```python
from build123d import *

# Parameters (mm, degrees)
SKETCH1_R           = 2.5
BOSS_EXTRUDE1_DEPTH = 3
SKETCH2_R           = 1.5
BOSS_EXTRUDE2_DEPTH = 30
CHAMFER1_SIZE       = 0.3
FILLET1_R           = 0.4
CUT_EXTRUDE1_DEPTH  = 1.5


with BuildPart() as part:
    # Sketch1 → Boss-Extrude1 (new body)
    with BuildSketch(Plane(origin=(0, 0, 0), x_dir=(1, 0, 0), z_dir=(0, 1, 0))):
        with Locations(Location((0, 0, 0), (0, 0, 270))):
            Circle(SKETCH1_R)
    extrude(amount=BOSS_EXTRUDE1_DEPTH)

    # Sketch2 → Boss-Extrude2 (add)
    with BuildSketch(Plane(origin=(0, 3, 0), x_dir=(1, 0, 0), z_dir=(0, 1, 0))):
        with Locations(Location((0, 0, 0), (0, 0, 270))):
            Circle(SKETCH2_R)
    extrude(amount=BOSS_EXTRUDE2_DEPTH)

    # Chamfer1
    chamfer1_edges = [part.edges().sort_by_distance(p)[0] for p in [
        (0, 33, -1.5),
    ]]
    chamfer(chamfer1_edges, length=CHAMFER1_SIZE)

    # Fillet1
    fillet1_edges = [part.edges().sort_by_distance(p)[0] for p in [
        (0, 0, -2.5),
        (0, 3, -2.5),
    ]]
    fillet(fillet1_edges, radius=FILLET1_R)

    # Sketch3 → Cut-Extrude1 (cut)
    with BuildSketch(Plane.XZ):
        Polygon((1.443375673, 0), (0.721687836, 1.25), (-0.721687836, 1.25), (-1.443375673, 0), (-0.721687836, -1.25), (0.721687836, -1.25), align=None)
    extrude(amount=-CUT_EXTRUDE1_DEPTH, mode=Mode.SUBTRACT)


solid = part.part
```
For this review, take the finished solid that the model builds, in its own axes (mm). A direction names the side the tool comes from. Coordinates: 2 decimals unless noted, no trailing zeros. Loops run counter-clockwise (first coordinate to the right, second up) from the corner with the lowest first, then second, coordinate; pieces in that order, holes last. Notation, with made-up numbers: (9.5, 40) - (64.5, 40) arc R23 ccw to (64.5, 53) - close; hole circle Ø7 at (29, 68). An arc over 180 degrees is marked (long way). Use one line per item in the form item = value. Start each with the question number.
1) Draft analysis for pull direction Z (two halves, no side actions). For faces 1 (the face through (-1.4, 3, 0.9)), 2 (the face through (0.45, 17.64, 1.43)), 3 (the face through (-1.08, 0.74, 0.63)), state which applies: released by +Z, released by -Z, zero draft, split by the parting line, or undercut.
2) Take a section at A-A (x = 0). State the section outline as (y, z) points, plus the area to 3 significant figures.
3) Take a section at B-B (y = 6.5). State the section outline as (x, z) points, plus the area to 3 significant figures.
4) For faces 4 (the face through (1.088, 0.74, 0.616)), 5 (the face through (0, 33, 0)), list the 3-axis set-ups (+Z, -Z, +X, -X, +Y, -Y) from which the entire face can be reached by the end or side of a thin tool; tool diameter is ignored.
5) To check wall thickness, follow probe 1 along Y at (x, z) = (0.8, -0.65); probe 2 along Y at (x, z) = (0.25, 2.05); probe 3 along X at (y, z) = (27.5, -0.9). State the ranges of each line that lie inside material, in increasing order. Write a range as from..to.
6) For pin 1 (2 mm diameter, centred on y = 13, z = -1.5, fed in from +X); pin 2 (2 mm diameter, centred on y = 14, z = -0.5, fed in from +X); pin 3 (2 mm diameter, centred on x = 0, y = 17, fed in from +Z), all flat-tipped, find the tip position at first contact; note any pin that passes through.
From the geometry:
q1.face_1 = zero draft
q1.face_2 = split by the parting line
q1.face_3 = undercut
q2.outline = (0, -2.1) arc R0.4 ccw to (0.4, -2.5) - (2.6, -2.5) arc R0.4 ccw to (3, -2.1) - (3, -1.5) - (32.7, -1.5) - (33, -1.2) - (33, 1.2) - (32.7, 1.5) - (3, 1.5) - (3, 2.1) arc R0.4 ccw to (2.6, 2.5) - (0.4, 2.5) arc R0.4 ccw to (0, 2.1) - (0, 1.25) - (1.5, 1.25) - (1.5, -1.25) - (0, -1.25) - close
q2.area = 101 mm2
q3.outline = circle Ø3 at (0, 0)
q3.area = 7.07 mm2
q4.face_4 = -Y
q4.face_5 = +Z, -Z, +X, -X, +Y
q5.probe_1 = 1.5..33
q5.probe_2 = 0..3
q5.probe_3 = -1.2..1.2
q6.pin_1 = 1.41
q6.pin_2 = 1.5
q6.pin_3 = 1.5
